Source: CAD feature listing. Evaluate the final solid. Frame: model axes, mm. Face numbers are marked on the shaded views. Give positions to 0.01 mm unless a question says otherwise; leave off trailing zeros. Write each loop counter-clockwise with the first axis right and the second up, starting at its lowest first coordinate (ties: lowest second). Pieces come first, ordered by that corner, then holes. Notation, with made-up numbers: (-2, -2.5) -> (15, -2.5) arc R31 ccw to (15, 25.5) -> close; hole circle Ø11 at (-30, 54.25). An arc over 180 degrees is marked (long way). Write item = value, one per line.
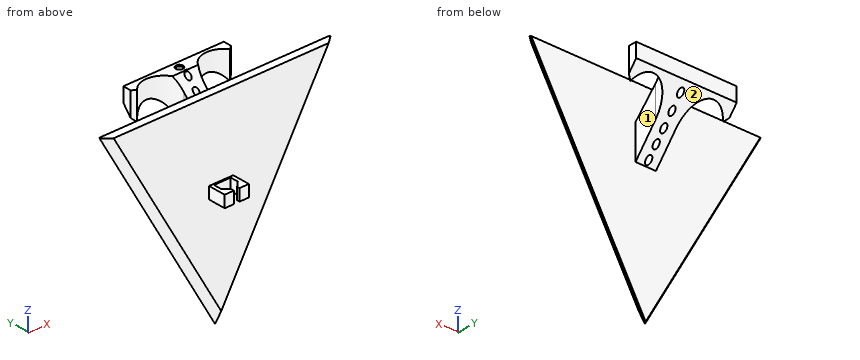
from build123d import *

# Parameters (mm, degrees)
BOSS_EXTRUDE1_DEPTH                       = 7.65
BOSS_EXTRUDE2_DEPTH                       = 5.08
CHAMFER1_SIZE                             = 1
CHAMFER2_SIZE                             = 1
CHAMFER3_SIZE                             = 5
CHAMFER4_SIZE                             = 5
BOSS_EXTRUDE3_DEPTH                       = 30
CUT_EXTRUDE1_DEPTH                        = 45.08
CUT_EXTRUDE3_DEPTH                        = 45.08
CUT_EXTRUDE4_DEPTH                        = 118.13273671
CUT_EXTRUDE4_DEPTH_BACK                   = 118.13273671
F_9_64_0_14063_DIAMETER_HOLE1_D           = 3.572002
F_9_64_0_14063_DIAMETER_HOLE1_CSINK_D     = 4.842002
F_9_64_0_14063_DIAMETER_HOLE1_CSINK_ANGLE = 100
CUT_EXTRUDE5_DEPTH                        = 118.132626096
CUT_EXTRUDE5_DEPTH_BACK                   = 118.132626096


with BuildPart() as part:
    # Sketch2 → Boss-Extrude1 (new body)
    with BuildSketch(Plane.XY):
        Polygon((-7.97490293, 0.58645445), (-7.97490293, -10.885302369), (-1.942800482, -10.885302369), (-1.942800482, -9.089251145), (-5.53490293, -5.497148696), (-5.53490293, -0.387148696), (-5.53490293, -0.287148696), (5.441404415, -0.287148696), (5.441404415, -0.387148696), (5.441404415, -5.497148696), (1.849301966, -9.089251145), (1.849301966, -10.885302369), (7.881404415, -10.885302369), (7.881404415, 0.58645445), align=None)
    extrude(amount=BOSS_EXTRUDE1_DEPTH)

    # Sketch3 → Boss-Extrude2 (add)
    with BuildSketch(Plane(origin=(0, 0.58645445, 0), x_dir=(1, 0, 0), z_dir=(0, 1, 0))):
        Polygon((-0.046749258, -58.45), (76.153250742, -58.45), (0, 76.2), (-76.246749258, -58.45), align=None)
    extrude(amount=BOSS_EXTRUDE2_DEPTH)

    # Chamfer1
    chamfer1_edges = [part.edges().sort_by_distance(p)[0] for p in [
        (38.076625371, 5.66645445, -8.875),
    ]]
    chamfer(chamfer1_edges, length=CHAMFER1_SIZE)

    # Chamfer2
    chamfer2_edges = [part.edges().sort_by_distance(p)[0] for p in [
        (-38.410764077, 5.66645445, -8.367476866),
    ]]
    chamfer(chamfer2_edges, length=CHAMFER2_SIZE)

    # Chamfer3
    # the kernel refuses this chamfer: 5 mm, written as the material it takes off along each edge
    with BuildSketch(Plane(origin=(6.335905635, 0.58645445, -87.389063167), x_dir=(-0.023926207208635007, 0.9996219169112968, -0.013548425709062981), z_dir=(-0.49274390851198024, 0, 0.8701743736885943))) as chamfer3_piece_1:
        Polygon((CHAMFER3_SIZE * 0.999621916911, -CHAMFER3_SIZE * 0.0274958766106), (-CHAMFER3_SIZE * 0.0274958766106, -CHAMFER3_SIZE * 0.999621916911), (0, 0), align=None)
    extrude(amount=180.455930537, mode=Mode.SUBTRACT)

    # Chamfer4
    # the kernel refuses this chamfer: 5 mm, written as the material it takes off along each edge
    with BuildSketch(Plane(origin=(82.483270671, 0.58645445, 69.642393956), x_dir=(-0.8701043132999969, -0.02749587661058631, 0.49210005156081454), z_dir=(-0.49228617663900415, 0, -0.870433409451953))) as chamfer4_piece_1:
        Polygon((CHAMFER4_SIZE * 0.999621916911, CHAMFER4_SIZE * 0.0274958766106), (-CHAMFER4_SIZE * 0.0274958766106, CHAMFER4_SIZE * 0.999621916911), (0, 0), align=None)
    extrude(amount=174.577450859, mode=Mode.SUBTRACT)

    # Sketch4 → Boss-Extrude3 (add)
    with BuildSketch(Plane(origin=(0, 5.66645445, 0), x_dir=(1, 0, 0), z_dir=(0, 1, 0))):
        Polygon((-7.97490293, -13.45), (7.881404415, -13.45), (32.881404415, -13.45), (32.881404415, -58.45), (7.881404415, -58.45), (-7.97490293, -58.45), (-32.97490293, -58.45), (-32.97490293, -13.45), align=None)
    extrude(amount=BOSS_EXTRUDE3_DEPTH)

    # Sketch5 → Cut-Extrude1 (cut)
    with BuildSketch(Plane(origin=(0, 0, 13.45), x_dir=(-1, 0, 0), z_dir=(0, 0, -1))):
        Polygon((-6.640745102, 5.66645445), (-32.881404415, 5.66645445), (-32.881404415, 30.285655528), (-6.640745102, 10.66645445), align=None)
        Polygon((6.734243618, 10.66645445), (6.734243618, 5.66645445), (32.97490293, 5.66645445), (32.97490293, 30.285655528), align=None)
    extrude(amount=-CUT_EXTRUDE1_DEPTH, mode=Mode.SUBTRACT)

    # Sketch7 → Cut-Extrude3 (cut)
    with BuildSketch(Plane(origin=(0, 0, 13.45), x_dir=(-1, 0, 0), z_dir=(0, 0, -1))):
        with BuildLine():
            Line((-6.640745102, 20.476054989), (-6.640745102, 10.66645445))
            Line((-6.640745102, 10.66645445), (-11.048165512, 10.66645445))
            ThreePointArc((-11.048165512, 10.66645445), (-31.728933629, 25.853173581), (-6.640745102, 20.476054989))
        make_face()
        with BuildLine():
            Line((6.734243618, 20.476054989), (6.734243618, 10.66645445))
            Line((6.734243618, 10.66645445), (11.141664027, 10.66645445))
            ThreePointArc((11.141664027, 10.66645445), (31.822432144, 25.853173581), (6.734243618, 20.476054989))
        make_face()
    extrude(amount=-CUT_EXTRUDE3_DEPTH, mode=Mode.SUBTRACT)

    # Sketch9 → Cut-Extrude4 (cut, two sides: drawn at the far end of the back side and taken through both)
    with BuildSketch(Plane.ZY.offset(6.734243618).offset(-CUT_EXTRUDE4_DEPTH_BACK)):
        Polygon((13.45, 5.66645445), (49.202607778, 35.66645445), (13.45, 35.66645445), align=None)
    extrude(amount=CUT_EXTRUDE4_DEPTH + CUT_EXTRUDE4_DEPTH_BACK, mode=Mode.SUBTRACT)

    # 9/64 (0.14063) Diameter Hole1 (through all)
    with Locations(Plane.XY.offset(58.45)):
        with Locations((0, 31.40818219), (0, 25.046150321), (0, 18.994461471), (0, 13.408287148), (0, 7.899698579)):
            CounterSinkHole(F_9_64_0_14063_DIAMETER_HOLE1_D / 2, F_9_64_0_14063_DIAMETER_HOLE1_CSINK_D / 2, counter_sink_angle=F_9_64_0_14063_DIAMETER_HOLE1_CSINK_ANGLE)

    # Sketch13 → Cut-Extrude5 (cut, two sides: drawn at the far end of the back side and taken through both)
    with BuildSketch(Plane(origin=(6.640745102, 0, 0), x_dir=(0, 0, -1), z_dir=(1, 0, 0)).offset(-CUT_EXTRUDE5_DEPTH_BACK)):
        Polygon((-58.45, 27.036219817), (-35.95, 5.66645445), (-58.45, 5.66645445), align=None)
    extrude(amount=CUT_EXTRUDE5_DEPTH + CUT_EXTRUDE5_DEPTH_BACK, mode=Mode.SUBTRACT)


solid = part.part
(1) Pull-direction query (Y, two-part tool) for the marked faces 1 and 2; classes: pulls with the +Y half, pulls with the -Y half, needs draft (parallel to the pull), parting line crosses it, or undercut.
Values follow:
face_1 = undercut
face_2 = pulls with the +Y half
(2) First-contact query: pin 1 (4 mm diameter, centred on x = 0, y = 7.9, fed in from +Z); pin 2 (12 mm diameter, centred on x = -24.5, z = 32, fed in from +Y); pin 3 (16.5 mm diameter, centred on y = 15, z = 30, fed in from +X); pin 4 (10 mm diameter, centred on y = 13, z = 4.5, fed in from -X). Flat tips, straight axial feed; report the tip coordinate or a pass-through.
Values follow:
pin_1 = 40.41
pin_2 = 5.67
pin_3 = 6.79
pin_4 = through
(3) Section query A-A (x = 11). Return loops of the section in (y, z), plus the area to 3 significant figures.
Values follow:
outline = (0.59, -46.59) -> (5.13, -55.82) -> (5.67, -54.72) -> (5.67, 58.45) -> (0.59, 58.45) -> close; (30.24, 42.74) -> (35.67, 49.2) -> (35.67, 58.45) -> (30.24, 58.45) -> close
area = 627 mm2
(4) Section query B-B (z = 2.5). Return loops of the section in (x, y), plus the area to 3 significant figures.
Values follow:
outline = (-44.04, 5.13) -> (-38.82, 0.59) -> (-7.97, 0.59) -> (-7.97, -10.89) -> (-1.94, -10.89) -> (-1.94, -9.09) -> (-5.53, -5.5) -> (-5.53, -0.29) -> (5.44, -0.29) -> (5.44, -5.5) -> (1.85, -9.09) -> (1.85, -10.89) -> (7.88, -10.89) -> (7.88, 0.59) -> (38.77, 0.59) -> (43.98, 5.13) -> (43.36, 5.67) -> (-43.42, 5.67) -> close
area = 514 mm2
(5) Section query C-C (z = -56). Return loops of the section in (x, y).
Values follow:
outline = (-10.91, 5.13) -> (-5.69, 0.59) -> (5.68, 0.59) -> (10.9, 5.13) -> (10.28, 5.67) -> (-10.29, 5.67) -> close
(6) Material intervals for line 1 (Y direction, x = 0, z = 29); line 2 (Y direction, x = 0, z = 45); line 3 (Y direction, x = 0, z = 32.75), sorted ascending.
Values follow:
line_1 = 0.59 to 6.11, 9.69 to 11.62, 15.19 to 17.21
line_2 = 0.59 to 5.67, 15.19 to 17.21, 20.78 to 23.26, 26.83 to 29.62
line_3 = 0.59 to 6.11, 9.69 to 11.62, 15.19 to 17.21, 20.78 to 21.86
